Model file for the job. Use its own axes, mm. Round coordinates to 2 decimals unless told otherwise and drop trailing zeros. Loops run counter-clockwise (first coordinate to the right, second up) from the corner with the lowest first, then second, coordinate; pieces in that order, holes last. Notation, with made-up numbers: (75.5, 30) -> (109.5, 30) arc R29 ccw to (109.5, 64) -> close; hole circle Ø4 at (8.25, -38). An arc over 180 degrees is marked (long way). Use a Markdown table: item, result.
Autodesk Inventor part; units mm, degrees
ref_plane "YZ Plane" through (0, 0, 0) normal (1, 0, 0) x (0, 1, 0)
ref_plane "XZ Plane" through (0, 0, 0) normal (0, 1, 0) x (-1, 0, 0)
ref_plane "XY Plane" through (0, 0, 0) normal (0, 0, 1) x (1, 0, 0)
sketch "Sketch1" plane through (0, 0, 0) normal (0, 0, 1) x (1, 0, 0)
  line L0 (-12.1708, 16.0073) -> (13.2292, 16.0073)
  line L1 (13.2292, 16.0073) -> (13.2292, -34.7927)
  line L2 (13.2292, -34.7927) -> (-12.1708, -34.7927)
  line L3 (-12.1708, -34.7927) -> (-12.1708, 16.0073)
  line L4 (11.9592, 14.7373) -> (-10.9008, 14.7373)
  line L5 (-10.9008, 14.7373) -> (-10.9008, -33.5227)
  line L6 (-10.9008, -33.5227) -> (11.9592, -33.5227)
  line L7 (11.9592, -33.5227) -> (11.9592, 14.7373)
  point P0 (0, 0)
  dimension "d0" = 25.4
  dimension "d1" = 50.8
  dimension "d2" = 1.27
extrude "Extrusion1" add sketch "Sketch1" along normal blind 444.5
sketch "Sketch2" plane through (-12.1708, 16.0073, 0) normal (0, 1, 0) x (1, 0, 0)
  circle A0 centre (12.7, -12.7) radius 1.7272
  line L0 (25.4, 0) -> (0, 0)
  line L1 (0, 0) -> (0, -444.5)
  point P0 (12.1708, 0)
  dimension "d5" = 3.4544
  dimension "d6" = 12.7
  dimension "d7" = 12.7
extrude "Extrusion2" cut sketch "Sketch2" against normal through all
pattern_linear "Rectangular Pattern1" count 44 spacing 25.4 along (0, 0, 1) of "Extrusion2"
equation "\"d3\" = d13"
equation "\"d10\" = d14"
equation "\"d13\" = 444.5"
equation "\"d14\" = d13"
equation "\"d32\" = 101.6"
properties part number "AIntakeSupport3"
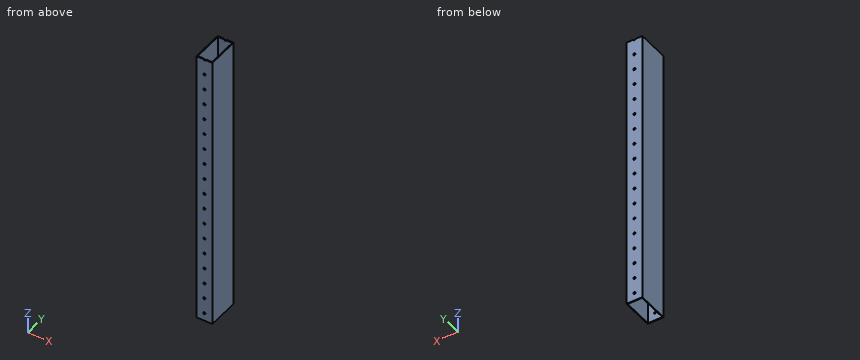
Q1. Flat gauge pins, fed straight in: pin 1 (5.5 mm diameter, centred on x = 0.53, z = 215.9, fed in from +Y); pin 2 (2 mm diameter, centred on x = 0.53, z = 368.3, fed in from -Y). Where does each tip first touch, or does it go through?
Results list:
| item | result |
|---|---|
| pin 1 | stops at y = 16.01 |
| pin 2 | passes through |
Q2. Drill centre lines: L1, parallel to X at y = 11, z = 205; L2, parallel to Y at x = 2.5, z = 248.5; L3, parallel to X at y = 15.5, z = 368.3. Where is each one in solid material? Low to high. Write a range as from..to.
Results list:
| item | result |
|---|---|
| L1 | x = -12.17..-10.9, 11.96..13.23 |
| L2 | y = -34.79..-33.52, 14.74..16.01 |
| L3 | x = -12.17..-1.2, 2.26..13.23 |
Q3. Band-saw the part on B-B, the plane y = -14. Give the cut face in (x, z), plus the area to 3 significant figures.
Results list:
| item | result |
|---|---|
| outline | (-12.17, 0) -> (-10.9, 0) -> (-10.9, 444.5) -> (-12.17, 444.5) -> close; (11.96, 0) -> (13.23, 0) -> (13.23, 444.5) -> (11.96, 444.5) -> close |
| area | 1,130 mm² |
Q4. Band-saw the part on A-A, the plane x = -6. Give the cut face in (y, z), plus the area to 3 significant figures.
Results list:
| item | result |
|---|---|
| outline | (-34.79, 0) -> (-33.52, 0) -> (-33.52, 444.5) -> (-34.79, 444.5) -> close; (14.74, 0) -> (16.01, 0) -> (16.01, 444.5) -> (14.74, 444.5) -> close |
| area | 1,130 mm² |
Q5. Band-saw the part on C-C, the plane z = 329.5. Give the cut face in (x, y), plus the area to 3 significant figures.
Results list:
| item | result |
|---|---|
| outline | (-12.17, -34.79) -> (13.23, -34.79) -> (13.23, 16.01) -> (-12.17, 16.01) -> close; hole (-10.9, -33.52) -> (11.96, -33.52) -> (11.96, 14.74) -> (-10.9, 14.74) -> close |
| area | 187 mm² |
